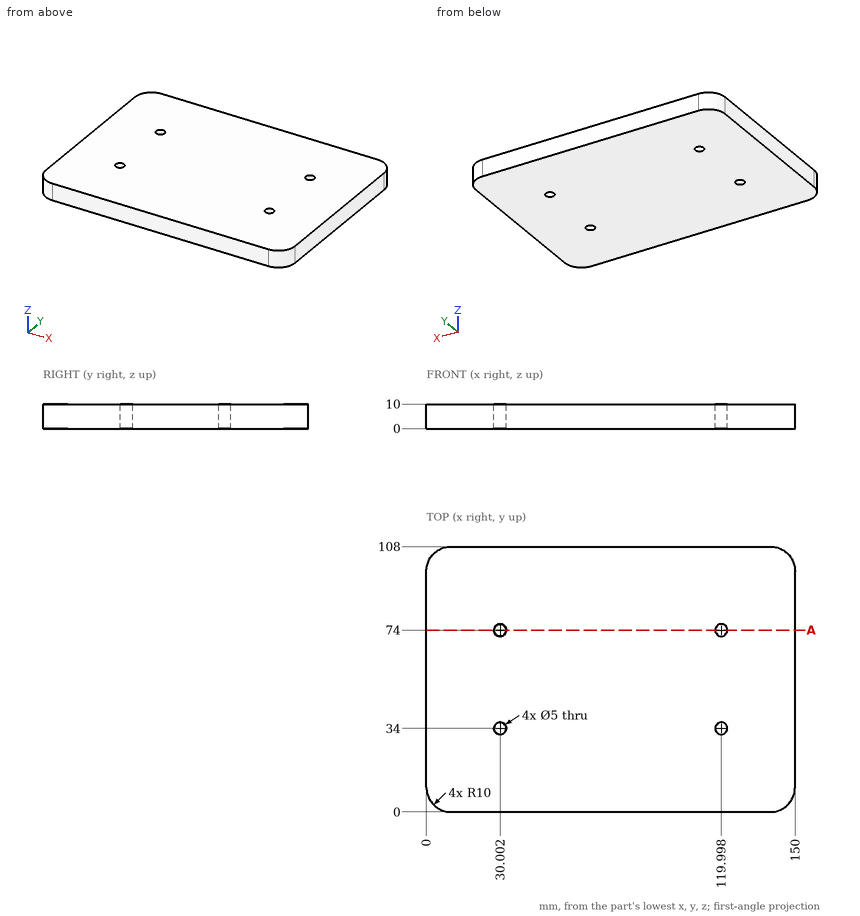
Answer from the drawing. Dimensions are ordinates in mm from the lowest x, y and z of the part. Coordinates: 2 decimals unless noted, no trailing zeros. Loops run counter-clockwise (first coordinate to the right, second up) from the corner with the lowest first, then second, coordinate; pieces in that order, holes last.
Q1. Each of these flat-tipped pins is pushed along its axis until it touches: pin 1 Ø2 at (y, z) = (45.5, 3) entering from -X; pin 2 Ø4.5 at (x, y) = (30, 34) entering from +Z. Where does it stop, or does it pass through?
Q2. Consider probe 1 along X at (y, z) = (74, 3.25). Determine where the line is inside the solid, lowest interval first.
Q3. The part is cut by section A-A on y = 74. Write down the section's boundary in (x, z), and give its area (3 significant figures).
Results below:
1. pin 1: stops at x = 0
1. pin 2: passes through
2. probe 1: x = 0 to 27.5, 32.5 to 117.5, 122.5 to 150
3. outline: (0, 0) - (27.5, 0) - (27.5, 10) - (0, 10) - close; (32.5, 0) - (117.5, 0) - (117.5, 10) - (32.5, 10) - close; (122.5, 0) - (150, 0) - (150, 10) - (122.5, 10) - close
3. area: 1,400 mm2
